```python
from build123d import *

# Parameters (mm, degrees)
SKETCH1_W           = 75
SKETCH1_H           = 35
BOSS_EXTRUDE1_DEPTH = 1
SKETCH2_R           = 1.5
SKETCH2_W           = 5
SKETCH2_H           = 20
CUT_EXTRUDE1_DEPTH  = 10
CHAMFER1_SIZE       = 2.5


with BuildPart() as part:
    # Sketch1 → Boss-Extrude1 (new body)
    with BuildSketch(Plane(origin=(0, 0, 0), x_dir=(1, 0, 0), z_dir=(0, 1, 0))):
        Rectangle(SKETCH1_W, SKETCH1_H)
    extrude(amount=BOSS_EXTRUDE1_DEPTH)

    # Sketch2 → Cut-Extrude1 (cut)
    with BuildSketch(Plane(origin=(0, 1, 0), x_dir=(1, 0, 0), z_dir=(0, 1, 0))):
        with Locations((22.5, 17.5)):
            Circle(SKETCH2_R)
        with Locations((22.5, -17.5)):
            Circle(SKETCH2_R)
        with Locations((-37.5, 0.89)):
            Rectangle(SKETCH2_W, SKETCH2_H)
    extrude(amount=-CUT_EXTRUDE1_DEPTH, mode=Mode.SUBTRACT)

    # Chamfer1
    chamfer1_edges = [part.edges().sort_by_distance(p)[0] for p in [
        (-35, 0.5, 9.11),
        (-35, 0.5, -10.89),
    ]]
    chamfer(chamfer1_edges, length=CHAMFER1_SIZE - 0.0001)  # a hair under: the kernel refuses the full size


solid = part.part
```
The model under review builds one solid part; all positions refer to its coordinate system, in mm. A direction names the side the tool comes from. Give positions to 0.01 mm unless a question says otherwise; leave off trailing zeros. Write each loop counter-clockwise with the first axis right and the second up, starting at its lowest first coordinate (ties: lowest second). Pieces come first, ordered by that corner, then holes. Notation, with made-up numbers: (-22.5, 12.25) -> (-1.5, 12.25) arc R19 ccw to (-1.5, 36.25) -> close; hole circle Ø2 at (26, 58). An arc over 180 degrees is marked (long way). Put each result on its own line as item: value.
(1) Tool access review of faces 5 (the flat face through (-1, 1, 0)), 6 (the flat face through (-36.23, 0.51, 7.84)): name each direction out of +Z, -Z, +X, -X, +Y, -Y from which nothing blocks a thin tool from reaching the whole face with its end or side.
Results are:
face 5: +Z, -Z, +X, -X, +Y
face 6: -X, +Y, -Y
(2) We need section B-B, the plane x = 22.5. Give the boundary of the cut face in (y, z), and give its area (3 significant figures).
Results are:
outline: (0, -16) -> (1, -16) -> (1, 16) -> (0, 16) -> close
area: 32.0 mm²
(3) The part is to be moulded in two halves that separate along X. For faces 1 (the cylindrical face through (22.5, 0.5, -16)), 2 (the flat face through (-36.27, 0.51, -9.66)), 3 (the cylindrical face through (22.5, 0.5, 16)), 4 (the flat face through (-1, 0, 0)), say which applies: pulls with the +X half, pulls with the -X half, needs draft (parallel to the pull), parting line crosses it, or undercut.
Results are:
face 1: undercut
face 2: pulls with the -X half
face 3: undercut
face 4: needs draft
(4) To check wall thickness, follow probe 1 along X at (y, z) = (0.55, 4.5); probe 2 along Z at (x, y) = (22.5, 0.3); probe 3 along X at (y, z) = (0.5, 7.5). State the ranges of each line that lie inside material, in increasing order. Write a range as from..to.
Results are:
probe 1: -35..37.5
probe 2: -16..16
probe 3: -35.89..37.5
